Job drawing, mm, ordinate dimensions from the low corner. One solid piece. Round coordinates to 2 decimals unless told otherwise and drop trailing zeros. Loops run counter-clockwise (first coordinate to the right, second up) from the corner with the lowest first, then second, coordinate; pieces in that order, holes last.
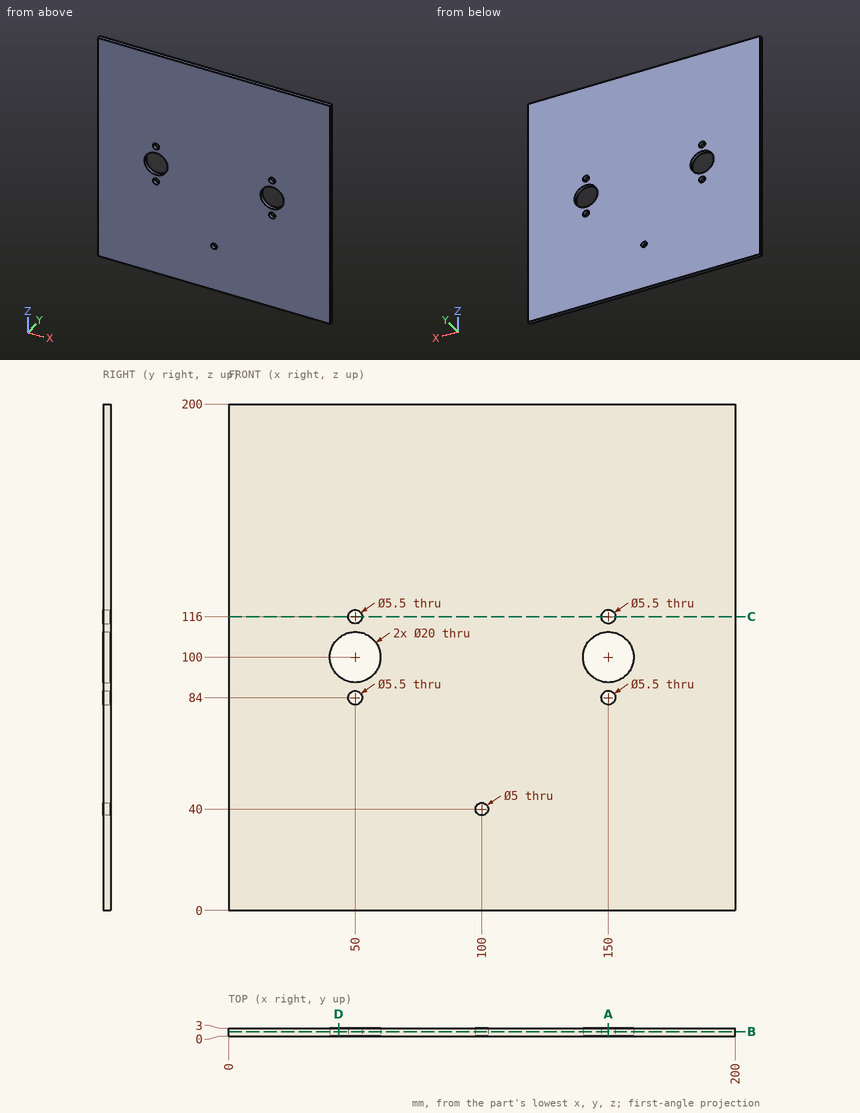
Item 1: Cut at A-A, the plane x = 150. Give the cut face in (y, z), plus the area to 3 significant figures.
Answers follow:
outline: (0, 0) - (3, 0) - (3, 81.25) - (0, 81.25) - close; (0, 86.75) - (3, 86.75) - (3, 90) - (0, 90) - close; (0, 110) - (3, 110) - (3, 113.25) - (0, 113.25) - close; (0, 118.75) - (3, 118.75) - (3, 200) - (0, 200) - close
area: 507 mm2
Item 2: Cut at B-B, the plane y = 1.75. Give the cut face in (x, z), plus the area to 3 significant figures.
Answers follow:
outline: (0, 0) - (200, 0) - (200, 200) - (0, 200) - close; hole circle Ø20 at (50, 100); hole circle Ø5.5 at (50, 84); hole circle Ø5.5 at (50, 116); hole circle Ø5 at (100, 40); hole circle Ø20 at (150, 100); hole circle Ø5.5 at (150, 84); hole circle Ø5.5 at (150, 116)
area: 39,300 mm2
Item 3: Cut at D-D, the plane x = 43.5. Give the cut face in (y, z), plus the area to 3 significant figures.
Answers follow:
outline: (0, 0) - (3, 0) - (3, 92.4) - (0, 92.4) - close; (0, 107.6) - (3, 107.6) - (3, 200) - (0, 200) - close
area: 554 mm2
Item 4: Cut at C-C, the plane z = 116. Give the cut face in (x, y), plus the area to 3 significant figures.
Answers follow:
outline: (0, 0) - (47.25, 0) - (47.25, 3) - (0, 3) - close; (52.75, 0) - (147.25, 0) - (147.25, 3) - (52.75, 3) - close; (152.75, 0) - (200, 0) - (200, 3) - (152.75, 3) - close
area: 567 mm2
Item 5: Probe line 1 (X direction, y = 2.45, z = 100); line 2 (Z direction, x = 50, y = 1.15); line 3 (X direction, y = 2.3, z = 84). List the from-to ranges inside material, lowest first.
Answers follow:
line 1: x = 0 to 40, 60 to 140, 160 to 200
line 2: z = 0 to 81.25, 86.75 to 90, 110 to 113.25, 118.75 to 200
line 3: x = 0 to 47.25, 52.75 to 147.25, 152.75 to 200
